Work out the finished part from the listing and answer in its coordinate system (mm). Face numbers are marked on the shaded views. A direction names the side the tool comes from. Coordinates: 2 decimals unless noted, no trailing zeros. Order: outer loops, then holes, each group sorted by start corner. A loop starts at its lowest first (then second) coordinate and runs counter-clockwise, first axis right, second up. Notation, with made-up numbers: M 21.5,83 L 44.5,83 A13 ccw 44.5,90 Z; hole C 15,83 d9. An arc over 180 degrees is marked long. Answer in a Markdown table with one row per item. Add a question column.
Item 1: Consider line 1 (Y direction, x = 14, z = 9.25); line 2 (X direction, y = 10.5, z = 8); line 3 (Z direction, x = 30, y = 10.5). Determine where each line is inside the solid, lowest interval first. Write a range as from..to.
Item 2: Flat-ended cylindrical pins translate along their axes: pin 1 Ø6 at (x, z) = (16, 9.5) entering from +Y; pin 2 Ø6 at (x, z) = (43.5, 4.5) entering from -Y; pin 3 Ø0.5 at (y, z) = (11.5, 10) entering from -X. Find the tip coordinate at first contact, or state that the pin passes through.
Item 3: The part is cut by section C-C (x = 43). Write down the section's boundary in (y, z).
Item 4: Which of the six approach directions +Z, -Z, +X, -X, +Y, -Y give full straight-line access (tool end or side, diameter ignored) to the marked faces 1, 2, 3 and 4?
Item 5: The mould has two halves that part along X. Classify the marked faces 5, 6, 7 and 8: released by +X, released by -X, zero draft, split by the parting line, or undercut.
Item 6: The part is cut by section A-A (y = 9.5). Write down the section's boundary in (x, z).
Item 7: The part is cut by section B-B (z = 4.75). Write down the section's boundary in (x, y), then the cut area to 3 significant figures.
Item 8: The part is cut by section D-D (y = 13). Write down the section's boundary in (x, z), then the cut area to 3 significant figures.
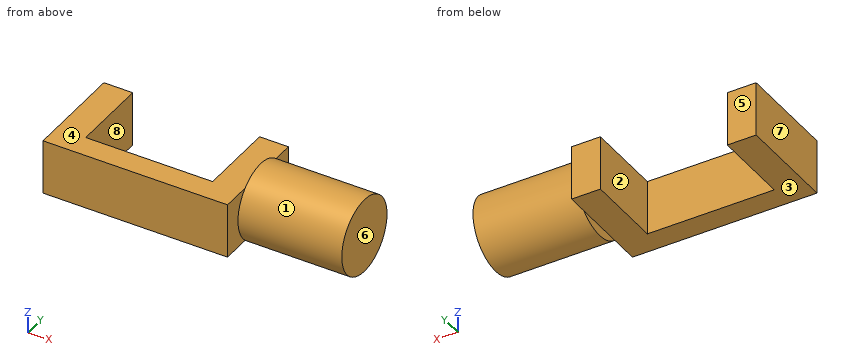
from build123d import *

# Parameters (mm, degrees)
SKETCH_1_W      = 32
SKETCH_1_H      = 9.5
EXTRUDE_1_DEPTH = 4
SKETCH_2_W      = 5
SKETCH_2_H      = 9.5
EXTRUDE_2_DEPTH = 13.5
SKETCH_3_W      = 5
SKETCH_3_H      = 9.5
EXTRUDE_3_DEPTH = 13.5
SKETCH_4_R      = 6.5
EXTRUDE_4_DEPTH = 18


with BuildPart() as part:
    # 草图1 → 凸台-拉伸1 (new body)
    with BuildSketch(Plane(origin=(0, 0, 0), x_dir=(1, 0, 0), z_dir=(0, 1, 0))):
        with Locations((16, -4.75)):
            Rectangle(SKETCH_1_W, SKETCH_1_H)
    extrude(amount=EXTRUDE_1_DEPTH)

    # 草图2 → 凸台-拉伸2 (add)
    with BuildSketch(Plane(origin=(0, 4, 0), x_dir=(1, 0, 0), z_dir=(0, 1, 0))):
        with Locations((2.5, -4.75)):
            Rectangle(SKETCH_2_W, SKETCH_2_H)
    extrude(amount=EXTRUDE_2_DEPTH)

    # 草图3 → 凸台-拉伸3 (add)
    with BuildSketch(Plane(origin=(0, 4, 0), x_dir=(1, 0, 0), z_dir=(0, 1, 0))):
        with Locations((29.5, -4.75)):
            Rectangle(SKETCH_3_W, SKETCH_3_H)
    extrude(amount=EXTRUDE_3_DEPTH)

    # 草图4 → 凸台-拉伸4 (add)
    with BuildSketch(Plane(origin=(32, 0, 0), x_dir=(0, 0, -1), z_dir=(1, 0, 0))):
        with Locations(Location((-4.75, 9.5, 0), (0, 0, 136.9509202))):
            Circle(SKETCH_4_R)
    extrude(amount=EXTRUDE_4_DEPTH)


solid = part.part
Reply:
| question | item | result |
|---|---|---|
| 1 | line 1 | y = 0..4 |
| 1 | line 2 | x = 0..5, 27..50 |
| 1 | line 3 | z = 0..9.5 |
| 2 | pin 1 | stops at y = 4 |
| 2 | pin 2 | stops at y = 3 |
| 2 | pin 3 | stops at x = 32 |
| 3 | outline | C 9.5,4.75 d13 |
| 4 | face 1 | +X |
| 4 | face 2 | +Z, -Z, +Y |
| 4 | face 3 | -Z, -X, +Y, -Y |
| 4 | face 4 | +Z, -X, +Y, -Y |
| 5 | face 5 | zero draft |
| 5 | face 6 | released by +X |
| 5 | face 7 | released by -X |
| 5 | face 8 | undercut |
| 6 | outline | M 0,0 L 5,0 L 5,9.5 L 0,9.5 Z; M 27,0 L 32,0 L 32,-1.75 L 50,-1.75 L 50,11.25 L 32,11.25 L 32,9.5 L 27,9.5 Z |
| 7 | outline | M 0,0 L 32,0 L 32,3 L 50,3 L 50,16 L 32,16 L 32,17.5 L 27,17.5 L 27,4 L 5,4 L 5,17.5 L 0,17.5 Z |
| 7 | area | 497 mm2 |
| 8 | outline | M 0,0 L 5,0 L 5,9.5 L 0,9.5 Z; M 27,0 L 32,0 L 32,-0.73 L 50,-0.73 L 50,10.23 L 32,10.23 L 32,9.5 L 27,9.5 Z |
| 8 | area | 292 mm2 |
